from build123d import *

# Parameters (mm, degrees)
SKETCH1_R           = 10
BOSS_EXTRUDE1_DEPTH = 400
CHAMFER1_SIZE       = 1
SKETCH2_R           = 3
CUT_EXTRUDE1_DEPTH  = 10
LPATTERN1_COUNT     = 3
LPATTERN1_PITCH     = 150


with BuildPart() as part:
    # Sketch1 → Boss-Extrude1 (new body)
    with BuildSketch(Plane.XY):
        Circle(SKETCH1_R)
    extrude(amount=BOSS_EXTRUDE1_DEPTH)

    # Chamfer1
    chamfer1_edges = [part.edges().sort_by_distance(p)[0] for p in [
        (-10, 0, 0),
        (-10, 0, 400),
    ]]
    chamfer(chamfer1_edges, length=CHAMFER1_SIZE)

    # Sketch2 → Cut-Extrude1 (cut)
    with BuildSketch(Plane(origin=(0, 0, 0), x_dir=(1, 0, 0), z_dir=(0, 1, 0))):
        with Locations((0, -15)):
            Circle(SKETCH2_R)
    cut_extrude1 = extrude(amount=-CUT_EXTRUDE1_DEPTH, mode=Mode.SUBTRACT)

    # LPattern1: Cut-Extrude1 ×3
    with Locations(*[(0, 0, i * LPATTERN1_PITCH) for i in range(1, LPATTERN1_COUNT)]):
        add(cut_extrude1, mode=Mode.SUBTRACT)


solid = part.part
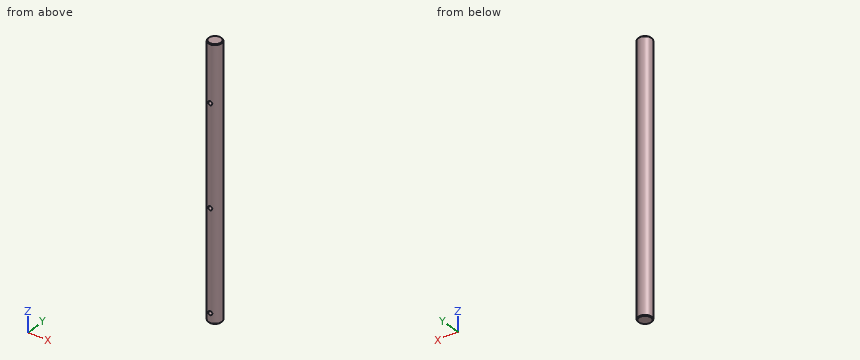
Could you check a few things on this model? Use its own coordinates, in mm. Coordinates: 2 decimals unless noted, no trailing zeros. Order: outer loops, then holes, each group sorted by start corner. A loop starts at its lowest first (then second) coordinate and runs counter-clockwise, first axis right, second up. Notation, with made-up numbers: (37.5, -13) -> (90.5, -13) arc R18 cw to (90.5, -7) -> close; hole circle Ø10 at (74.5, -24). An arc over 180 degrees is marked (long way). One line per item, written item: value. Start each with the question number.
1) I'm going to push flat-ended pins straight in: pin 1 (5 mm diameter, centred on x = 0, z = 165, fed in from -Y); pin 2 (6 mm diameter, centred on x = -6.5, z = 245, fed in from -Y); pin 3 (3 mm diameter, centred on x = -2.5, z = 279.5, fed in from -Y). Where does each tip first touch, or does it pass through?
2) If I drill on L1, parallel to Z at x = 0, y = -8; L2, parallel to Y at x = 0.5, z = 230; L3, parallel to X at y = -6.5, z = 15, over which ranges is the centre line in solid material (lowest first)? Write a range as [from, to].
3) Imagine slicing it at A-A on z = 253. List the corners of the cut face in (x, y) for me, plus the area to 3 significant figures.
Answer list:
1. pin 1: stops at y = 0
1. pin 2: stops at y = -9.37
1. pin 3: stops at y = -9.95
2. L1: z = [0, 12], [18, 162], [168, 312], [318, 400]
2. L2: y = [-9.99, 9.99]
2. L3: x = [-7.6, -3], [3, 7.6]
3. outline: circle Ø20 at (0, 0)
3. area: 314 mm2
